Read the model definition and answer for the solid it produces. Units are mm, in the model's axes. Face numbers are marked on the shaded views. A direction names the side the tool comes from. Round coordinates to 2 decimals unless told otherwise and drop trailing zeros. Order: outer loops, then holes, each group sorted by start corner. A loop starts at its lowest first (then second) coordinate and runs counter-clockwise, first axis right, second up. Notation, with made-up numbers: (-16, 70.25) -> (0, 70.25) arc R13 ccw to (0, 80.25) -> close; hole circle Ø2 at (-15, 19.5). An arc over 180 degrees is marked (long way). One line per item, written item: value. Start each with the question number.
1. Consider line 1 (Z direction, x = 2.5, y = -6.5); line 2 (Z direction, x = -4, y = -3.75); line 3 (Y direction, x = -4, z = -42.5). Determine where each line is inside the solid, lowest interval first.
2. Section B-B (x = 0) is taken. Give the vertices of the cut face in (y, z).
3. For the marked faces 1 and 2, determine the directions among +Z, -Z, +X, -X, +Y, -Y from which every point of the face is accessible in a straight line to the end or side of a thin tool.
4. Section C-C (z = -23) is taken. Give the vertices of the cut face in (x, y), then the cut area to 3 significant figures.
5. Flat-ended cylindrical pins translate along their axes: pin 1 Ø5 at (x, z) = (0, -3) entering from +Y; pin 2 Ø3 at (x, z) = (1, -47) entering from -Y; pin 3 Ø2.5 at (x, z) = (-0.5, -3.5) entering from -Y. Find the tip coordinate at first contact, or state that the pin passes through.
6. Section A-A (y = 0) is taken. Give the vertices of the cut face in (x, z).
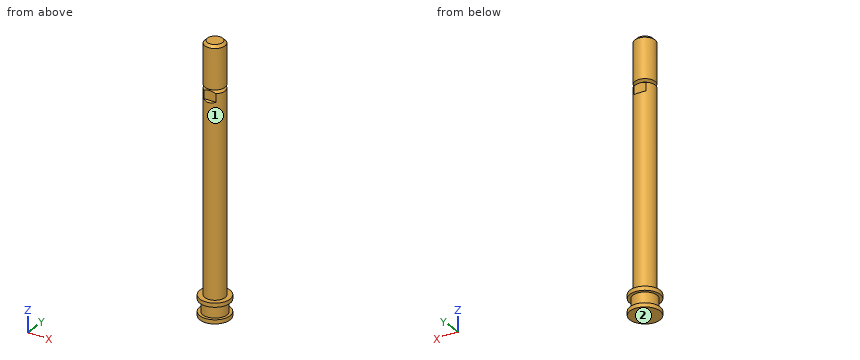
from build123d import *

# Parameters (mm, degrees)
SMUSSO1_SIZE                  = 1.25
TAGLIO_ESTRUSIONE1_DEPTH      = 8.5
TAGLIO_ESTRUSIONE1_DEPTH_BACK = 8.5


with BuildPart() as part:
    # Schizzo1 → Rivoluzione1 (revolve)
    with BuildSketch(Plane(origin=(0, 0, 0), x_dir=(0, 0, -1), z_dir=(1, 0, 0))):
        Polygon((0, 0), (-22, 0), (-22, 5), (-0.866025404, 5), (0, 3.5), (0.866025404, 5), (100, 5), (100, 7.5), (102, 7.5), (102, 6), (108, 6), (108, 7.5), (110, 7.5), (110, 0), align=None)
    revolve(axis=Axis((0, 0, 22), (0, 0, 1)))

    # Smusso1
    smusso1_edges = [part.edges().sort_by_distance(p)[0] for p in [
        (0, -5, 22),
    ]]
    chamfer(smusso1_edges, length=SMUSSO1_SIZE)

    # Schizzo2 → Taglio-Estrusione1 (cut, two sides)
    with BuildSketch(Plane(origin=(0, 0, 0), x_dir=(0, 0, -1), z_dir=(1, 0, 0))) as taglio_estrusione1_sk:
        Polygon((5.577350269, 5), (0, 5), (0, 4), (5, 4), align=None)
        Polygon((0, -5), (0, -4), (5, -4), (5.577350269, -5), align=None)
    extrude(amount=TAGLIO_ESTRUSIONE1_DEPTH, mode=Mode.SUBTRACT)
    extrude(taglio_estrusione1_sk.sketch, amount=-TAGLIO_ESTRUSIONE1_DEPTH_BACK, mode=Mode.SUBTRACT)


solid = part.part
Answer:
1. line 1: -110 to -108, -102 to -100
1. line 2: -110 to -100
1. line 3: -3 to 3
2. outline: (-7.5, -110) -> (7.5, -110) -> (7.5, -108) -> (6, -108) -> (6, -102) -> (7.5, -102) -> (7.5, -100) -> (5, -100) -> (5, -5.58) -> (4, -5) -> (4, -0.29) -> (3.5, 0) -> (5, 0.87) -> (5, 20.75) -> (3.75, 22) -> (-3.75, 22) -> (-5, 20.75) -> (-5, 0.87) -> (-3.5, 0) -> (-4, -0.29) -> (-4, -5) -> (-5, -5.58) -> (-5, -100) -> (-7.5, -100) -> (-7.5, -102) -> (-6, -102) -> (-6, -108) -> (-7.5, -108) -> close
3. face 1: +Z
3. face 2: -Z, +X, -X, +Y, -Y
4. outline: circle Ø10 at (0, 0)
4. area: 78.5 mm^2
5. pin 1: y = 4.87
5. pin 2: y = -5
5. pin 3: y = -4
6. outline: (-7.5, -110) -> (7.5, -110) -> (7.5, -108) -> (6, -108) -> (6, -102) -> (7.5, -102) -> (7.5, -100) -> (5, -100) -> (5, -0.87) -> (3.5, 0) -> (5, 0.87) -> (5, 20.75) -> (3.75, 22) -> (-3.75, 22) -> (-5, 20.75) -> (-5, 0.87) -> (-3.5, 0) -> (-5, -0.87) -> (-5, -100) -> (-7.5, -100) -> (-7.5, -102) -> (-6, -102) -> (-6, -108) -> (-7.5, -108) -> close
